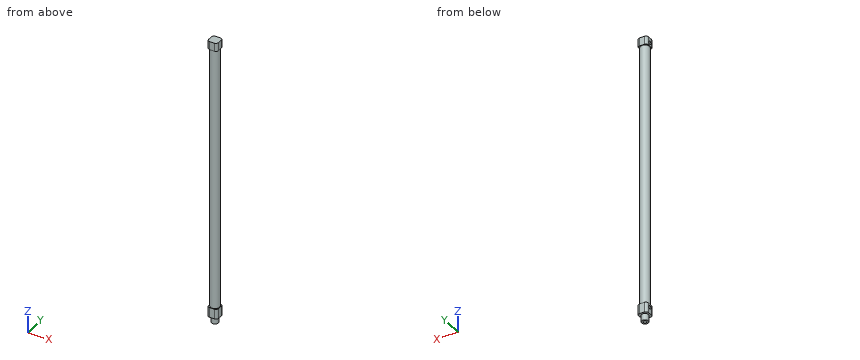
```python
from build123d import *

# Parameters (mm, degrees)
SKETCH_1_R          = 5.5
SKETCH_1_R_2        = 5
EXTRUDE_1_DEPTH     = 320
EXTRUDE_2_DEPTH     = 10
EXTRUDE_3_DEPTH     = 12
SKETCH_4_R          = 4
EXTRUDE_4_DEPTH     = 8
SKETCH_5_R          = 2
CUT_EXTRUDE_1_DEPTH = 38
SKETCH_6_R          = 2
CUT_EXTRUDE_3_DEPTH = 3


with BuildPart() as part:
    # 草图1 → 凸台-拉伸1 (new body)
    with BuildSketch(Plane.XY):
        Circle(SKETCH_1_R)
        Circle(SKETCH_1_R_2, mode=Mode.SUBTRACT)
    extrude(amount=EXTRUDE_1_DEPTH)

    # 草图2 → 凸台-拉伸2 (add)
    with BuildSketch(Plane.XY.offset(320)):
        with BuildLine():
            Line((-3, -6), (3, -6))
            ThreePointArc((3, -6), (5.121320344, -5.121320344), (6, -3))
            Line((6, -3), (6, 3))
            ThreePointArc((6, 3), (5.121320344, 5.121320344), (3, 6))
            Line((3, 6), (-3, 6))
            ThreePointArc((-3, 6), (-5.121320344, 5.121320344), (-6, 3))
            Line((-6, 3), (-6, -3))
            ThreePointArc((-6, -3), (-5.121320344, -5.121320344), (-3, -6))
        make_face()
    extrude(amount=EXTRUDE_2_DEPTH)

    # 草图3 → 凸台-拉伸3 (add)
    with BuildSketch(Plane(origin=(0, 0, 0), x_dir=(-1, 0, 0), z_dir=(0, 0, -1))):
        with BuildLine():
            Line((-3, -6), (3, -6))
            ThreePointArc((3, -6), (5.121320344, -5.121320344), (6, -3))
            Line((6, -3), (6, 3))
            ThreePointArc((6, 3), (5.121320344, 5.121320344), (3, 6))
            Line((3, 6), (-3, 6))
            ThreePointArc((-3, 6), (-5.121320344, 5.121320344), (-6, 3))
            Line((-6, 3), (-6, -3))
            ThreePointArc((-6, -3), (-5.121320344, -5.121320344), (-3, -6))
        make_face()
    extrude(amount=EXTRUDE_3_DEPTH)

    # 草图4 → 凸台-拉伸4 (add)
    with BuildSketch(Plane(origin=(0, 0, -12), x_dir=(-1, 0, 0), z_dir=(0, 0, -1))):
        Circle(SKETCH_4_R)
    extrude(amount=EXTRUDE_4_DEPTH)

    # 草图5 → 切除-拉伸1 (cut)
    with BuildSketch(Plane(origin=(0, 0, -20), x_dir=(-1, 0, 0), z_dir=(0, 0, -1))):
        Circle(SKETCH_5_R)
    extrude(amount=-CUT_EXTRUDE_1_DEPTH, mode=Mode.SUBTRACT)

    # 草图6 → 切除-拉伸3 (cut)
    with BuildSketch(Plane.ZY.offset(6)):
        with Locations((-4, 0)):
            Circle(SKETCH_6_R)
        with Locations((324, 0)):
            Circle(SKETCH_6_R)
    extrude(amount=-CUT_EXTRUDE_3_DEPTH, mode=Mode.SUBTRACT)


solid = part.part
```
Geometry: final body of the model. Coordinates: model frame, mm. Round coordinates to 2 decimals unless told otherwise and drop trailing zeros. Write each loop counter-clockwise with the first axis right and the second up, starting at its lowest first coordinate (ties: lowest second). Pieces come first, ordered by that corner, then holes. Notation, with made-up numbers: M 50,25 L 101,25 A26 ccw 101,51 Z; hole C 76,34.5 d8. An arc over 180 degrees is marked long. Answer in a Markdown table with one row per item. Add a question column.
(1) Contact query for flat-ended pins moving along their axis: pin 1 (3 mm diameter, centred on x = 4.5, y = -3.5, fed in from -Z); pin 2 (5 mm diameter, centred on y = -3, z = 97.5, fed in from -X); pin 3 (1.5 mm diameter, centred on x = 1.5, z = 86, fed in from -Y). Output: stop coordinate, or through.
(2) Ray query, L1, parallel to Z at x = -3.75, y = 0.5; L2, parallel to Z at x = -1.75, y = 1.75; L3, parallel to Z at x = 3.5, y = -5. Return the intervals inside material, ascending.
(3) Cut plane A-A, the plane z = 62. Return the cut outline in (x, y).
Established:
| question | item | result |
|---|---|---|
| 1 | pin 1 | z = -12 |
| 1 | pin 2 | x = -5.48 |
| 1 | pin 3 | y = -5.45 |
| 2 | L1 | -20 to -5.94, -2.06 to 0, 320 to 322.06, 325.94 to 330 |
| 2 | L2 | -20 to 0, 320 to 330 |
| 2 | L3 | -12 to 0, 320 to 330 |
| 3 | outline | C 0,0 d11; hole C 0,0 d10 |
